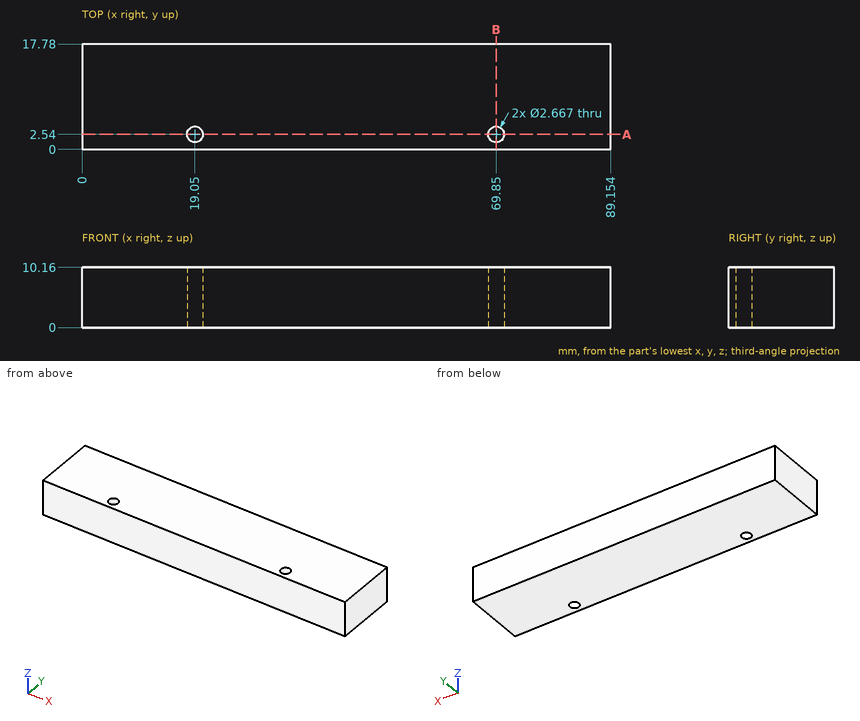
For this review, use the dimensioned drawing (mm, ordinates from the lowest corner) and the shaded views. Coordinates: 2 decimals unless noted, no trailing zeros. Write each loop counter-clockwise with the first axis right and the second up, starting at its lowest first coordinate (ties: lowest second). Pieces come first, ordered by that corner, then holes. Notation, with made-up numbers: (64, -32) - (123, -32) arc R15 cw to (123, -11) - close; hole circle Ø2 at (82.5, 15). An arc over 180 degrees is marked (long way). Answer in a Markdown table with one row per item. Add a question column.
Q1. Consider section B-B on x = 69.85. Give the boundary of the cut face in (y, z).
Q2. Clearance check with a flat-ended pin moving along its axis: pin 1 (1.6 mm diameter, centred on x = 69.85, y = 2.54, fed in from -Z). State where the tip first meets the part, or that it passes through.
Q3. To check wall thickness, follow line 1 along X through (y, z) = (2.54, 3.25); line 2 along Y through (x, z) = (19.05, 6.75); line 3 along X through (y, z) = (3.25, 5.5). State the ranges of each line that lie inside material, in increasing order. Write a range as from..to.
Q4. Consider section A-A on y = 2.54. Give the boundary of the cut face in (x, z).
Answers below:
| question | item | result |
|---|---|---|
| 1 | outline | (0, 0) - (1.21, 0) - (1.21, 10.16) - (0, 10.16) - close; (3.87, 0) - (17.78, 0) - (17.78, 10.16) - (3.87, 10.16) - close |
| 2 | pin 1 | through |
| 3 | line 1 | 0..17.72, 20.38..68.52, 71.18..89.15 |
| 3 | line 2 | 0..1.21, 3.87..17.78 |
| 3 | line 3 | 0..17.92, 20.18..68.72, 70.98..89.15 |
| 4 | outline | (0, 0) - (17.72, 0) - (17.72, 10.16) - (0, 10.16) - close; (20.38, 0) - (68.52, 0) - (68.52, 10.16) - (20.38, 10.16) - close; (71.18, 0) - (89.15, 0) - (89.15, 10.16) - (71.18, 10.16) - close |
